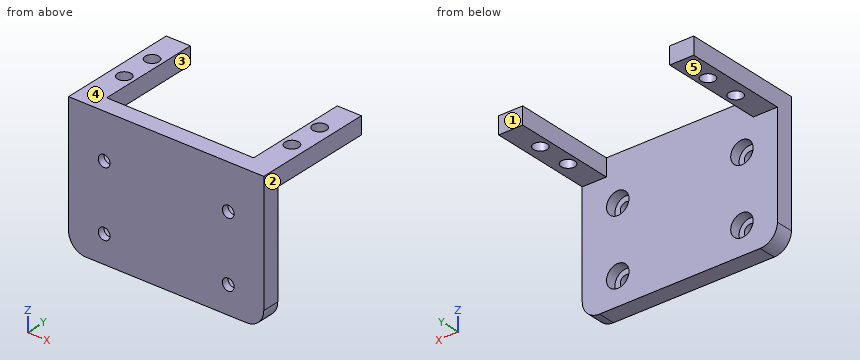
```python
from build123d import *

# Parameters (mm, degrees)
SKETCH3_W                      = 56.6
SKETCH3_H                      = 40
BOSS_EXTRUDE1_DEPTH            = 5
SKETCH2_W                      = 7
SKETCH2_H                      = 29.9
SKETCH2_R                      = 2
BOSS_EXTRUDE2_DEPTH            = 5
CBORE_FOR_M3_SHCS2_D           = 3.4
CBORE_FOR_M3_SHCS2_DEPTH       = 5
CBORE_FOR_M3_SHCS2_CBORE_D     = 6.5
CBORE_FOR_M3_SHCS2_CBORE_DEPTH = 3
CBORE_FOR_M3_SHCS2_TIP         = 1.021463052
FILLET1_R                      = 5


with BuildPart() as part:
    # Sketch3 → Boss-Extrude1 (new body)
    with BuildSketch(Plane(origin=(0, 0, 0), x_dir=(1, 0, 0), z_dir=(0, 1, 0))):
        with Locations((0, 20)):
            Rectangle(SKETCH3_W, SKETCH3_H)
    extrude(amount=-BOSS_EXTRUDE1_DEPTH)

    # Sketch2 → Boss-Extrude2 (add)
    # profile 1 of 2: a face of its own
    with BuildSketch(Plane.XY):
        with Locations((-24.8, 14.95)):
            Rectangle(SKETCH2_W, SKETCH2_H)
        with Locations((-24.3, 19.9)):
            Circle(SKETCH2_R, mode=Mode.SUBTRACT)
        with Locations((-24.3, 10)):
            Circle(SKETCH2_R, mode=Mode.SUBTRACT)
    # profile 2 of 2: a face of its own
    with BuildSketch(Plane.XY):
        with Locations((24.8, 14.95)):
            Rectangle(SKETCH2_W, SKETCH2_H)
        with Locations(Location((24.3, 10, 0), (0, 0, 180))):
            Circle(SKETCH2_R, mode=Mode.SUBTRACT)
        with Locations(Location((24.3, 19.9, 0), (0, 0, 180))):
            Circle(SKETCH2_R, mode=Mode.SUBTRACT)
    extrude(amount=-BOSS_EXTRUDE2_DEPTH)

    # CBORE for M3 SHCS2
    with Locations(Plane(origin=(0, 0, 0), x_dir=(1, 0, 0), z_dir=(0, 1, 0))):
        with Locations((-18, 32), (18, 13), (-18, 13), (18, 32)):
            CounterBoreHole(CBORE_FOR_M3_SHCS2_D / 2, CBORE_FOR_M3_SHCS2_CBORE_D / 2, CBORE_FOR_M3_SHCS2_CBORE_DEPTH, depth=CBORE_FOR_M3_SHCS2_DEPTH)
            with Locations((0, 0, -(CBORE_FOR_M3_SHCS2_DEPTH + CBORE_FOR_M3_SHCS2_TIP / 2))):  # 118° drill point
                Cone(0, CBORE_FOR_M3_SHCS2_D / 2, CBORE_FOR_M3_SHCS2_TIP, mode=Mode.SUBTRACT)

    # Fillet1
    fillet1_edges = [part.edges().sort_by_distance(p)[0] for p in [
        (-28.3, -2.5, -40),
        (28.3, -2.5, -40),
    ]]
    fillet(fillet1_edges, radius=FILLET1_R)


solid = part.part
```
Geometry check sheet. Reference: the model listing, model coordinates, mm. Face numbers are marked on the shaded views. A direction names the side the tool comes from. Coordinates: 2 decimals unless noted, no trailing zeros. Order: outer loops, then holes, each group sorted by start corner. A loop starts at its lowest first (then second) coordinate and runs counter-clockwise, first axis right, second up.
Item 1: Scan lines: line 1 along Z through (x, y) = (18, -4.5); line 2 along Z through (x, y) = (-18, -2); line 3 along X through (y, z) = (-2.2, -32). Record each from-to range of solid material in increasing order.
Item 2: Section check C-C (x = 18). Enter the section's corners in (y, z), plus the area to 3 significant figures.
Item 3: Section check A-A (y = 5.5). Enter the section's corners in (x, z), plus the area to 3 significant figures.
Item 4: Section check B-B (z = -13). Enter the section's corners in (x, y), plus the area to 3 significant figures.
Item 5: Section check D-D (y = 10). Enter the section's corners in (x, z).
Item 6: Tool access check on the marked faces 4 and 5. Record the directions out of +Z, -Z, +X, -X, +Y, -Y that give a thin tool (end or side, any length) a straight path to the whole face; none if there is none.
Item 7: Depth check by flat-ended pin: pin 1 (5 mm diameter, centred on x = 17, z = -33, fed in from +Y); pin 2 (2.5 mm diameter, centred on x = 18, z = -13, fed in from -Y); pin 3 (5.5 mm diameter, centred on x = -24.5, y = 7.5, fed in from -Z); pin 4 (2 mm diameter, centred on x = 16.5, z = -13.5, fed in from +Y). Enter the tip coordinate at first touch or a pass-through.
Item 8: Mould release check, pull along X, two halves, no side actions. Record for the marked faces 1, 2 and 3: released by +X, released by -X, zero draft, split by the parting line, or undercut.
Check sheet entries:
1. line 1: z = -40 to -33.7, -30.3 to -14.7, -11.3 to 0
1. line 2: z = -40 to -35.25, -28.75 to -16.25, -9.75 to 0
1. line 3: x = -28.3 to -21.25, -14.75 to 14.75, 21.25 to 28.3
2. outline: (-5, -40) - (0, -40) - (0, -35.25) - (-3, -35.25) - (-3, -33.7) - (-5, -33.7) - close; (-5, -30.3) - (-3, -30.3) - (-3, -28.75) - (0, -28.75) - (0, -16.25) - (-3, -16.25) - (-3, -14.7) - (-5, -14.7) - close; (-5, -11.3) - (-3, -11.3) - (-3, -9.75) - (0, -9.75) - (0, 0) - (-5, 0) - close
2. area: 147 mm2
3. outline: (-28.3, -5) - (-21.3, -5) - (-21.3, 0) - (-28.3, 0) - close; (21.3, -5) - (28.3, -5) - (28.3, 0) - (21.3, 0) - close
3. area: 70.0 mm2
4. outline: (-28.3, -5) - (-19.7, -5) - (-19.7, -3) - (-21.25, -3) - (-21.25, 0) - (-28.3, 0) - close; (-16.3, -5) - (16.3, -5) - (16.3, -3) - (14.75, -3) - (14.75, 0) - (-14.75, 0) - (-14.75, -3) - (-16.3, -3) - close; (19.7, -5) - (28.3, -5) - (28.3, 0) - (21.25, 0) - (21.25, -3) - (19.7, -3) - close
4. area: 230 mm2
5. outline: (-28.3, -5) - (-26.3, -5) - (-26.3, 0) - (-28.3, 0) - close; (-22.3, -5) - (-21.3, -5) - (-21.3, 0) - (-22.3, 0) - close; (21.3, -5) - (22.3, -5) - (22.3, 0) - (21.3, 0) - close; (26.3, -5) - (28.3, -5) - (28.3, 0) - (26.3, 0) - close
6. face 4: +Z, +X, -X, +Y, -Y
6. face 5: -Z, +X, -X, +Y
7. pin 1: stops at y = 0
7. pin 2: passes through
7. pin 3: stops at z = -5
7. pin 4: stops at y = -3
8. face 1: zero draft
8. face 2: released by +X
8. face 3: undercut
